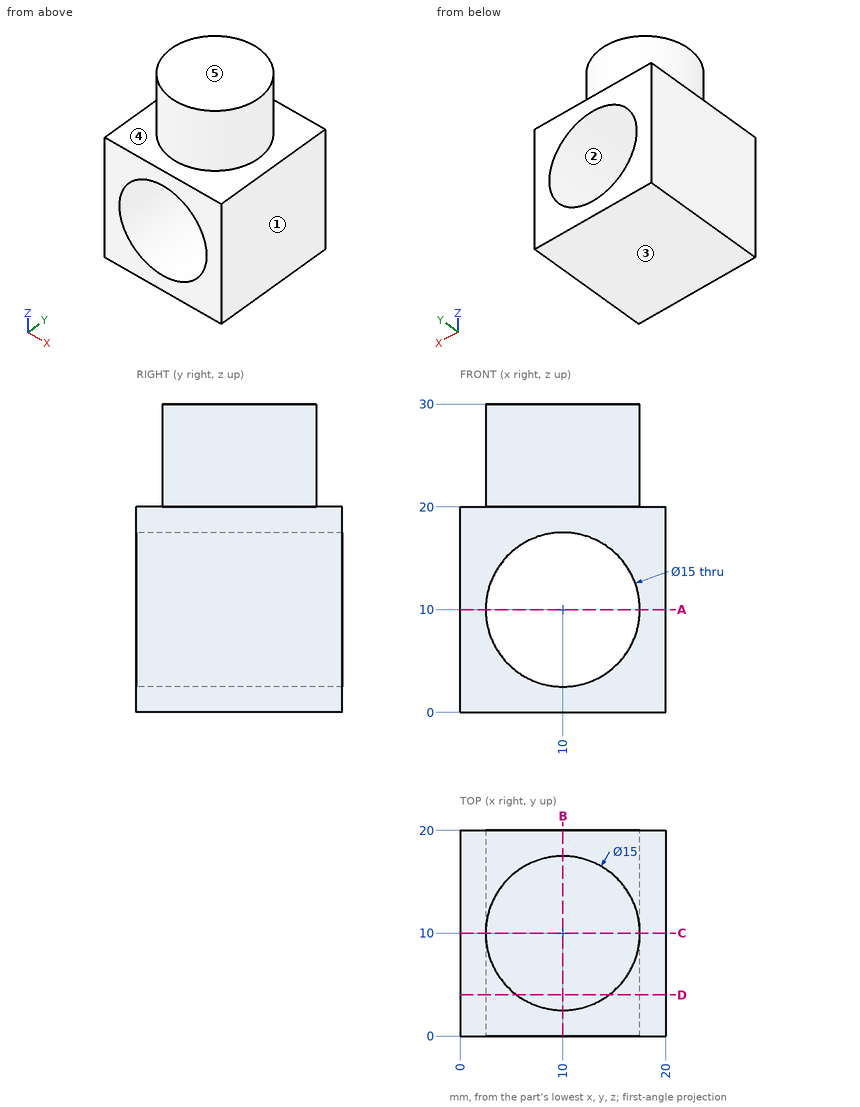
Verification items for this drawing (mm, ordinates from the low corner). A direction names the side the tool comes from. Give positions to 0.01 mm unless a question says otherwise; leave off trailing zeros. Loops run counter-clockwise (first coordinate to the right, second up) from the corner with the lowest first, then second, coordinate; pieces in that order, holes last. Notation, with made-up numbers: M 6.5,-30 L 24.5,-30 A21 ccw 24.5,8 Z; hole C 24.25,79.5 d4. An arc over 180 degrees is marked long. Answer as a JSON object with one key per item and string values. Group by question number.
Q1. Release check for a two-part mould opening along X. For the marked faces 1, 2 and 3 record: released by +X, released by -X, zero draft, split by the parting line, or undercut.
Q2. Cross-section at A-A on z = 10. Record the cut outline in (x, y), then the cut area to 3 significant figures.
Q3. Access from +Z, -Z, +X, -X, +Y, -Y to the whole of each face (thin tool, end or side, straight path). Record for the marked faces 4 and 5.
Q4. Material ranges on line 1 along Z through (x, y) = (10, 11.25); line 2 along Z through (x, y) = (1.5, 16); line 3 along Z through (x, y) = (5.5, 1.5), recorded low to high. Write a range as [from, to].
Q5. Cross-section at D-D on y = 4. Record the cut outline in (x, z).
Q6. Cross-section at B-B on x = 10. Record the cut outline in (y, z), then the cut area to 3 significant figures.
Q7. Cross-section at C-C on y = 10. Record the cut outline in (x, z), then the cut area to 3 significant figures.
Evaluation:
{
 "1": {"face 1": "released by +X", "face 2": "undercut", "face 3": "zero draft"},
 "2": {"outline": "M 0,0 L 2.5,0 L 2.5,20 L 0,20 Z; M 17.5,0 L 20,0 L 20,20 L 17.5,20 Z", "area": "100 mm2"},
 "3": {"face 4": "+Z", "face 5": "+Z, +X, -X, +Y, -Y"},
 "4": {"line 1": "z = [0, 2.5], [17.5, 30]", "line 2": "z = [0, 20]", "line 3": "z = [0, 4], [16, 20]"},
 "5": {"outline": "M 0,0 L 20,0 L 20,20 L 14.5,20 L 14.5,30 L 5.5,30 L 5.5,20 L 0,20 Z; hole C 10,10 d15"},
 "6": {"outline": "M 0,0 L 20,0 L 20,2.5 L 0,2.5 Z; M 0,17.5 L 20,17.5 L 20,20 L 17.5,20 L 17.5,30 L 2.5,30 L 2.5,20 L 0,20 Z", "area": "250 mm2"},
 "7": {"outline": "M 0,0 L 20,0 L 20,20 L 17.5,20 L 17.5,30 L 2.5,30 L 2.5,20 L 0,20 Z; hole C 10,10 d15", "area": "373 mm2"}
}
